```python
from build123d import *

# Parameters (mm, degrees)
F1_DEPTH = 6
F5_DEPTH = 9
F2_R     = 2.05
F6_DEPTH = 13
F2_R_2   = 3.5
F7_DEPTH = 2
F8_DEPTH = 2
F9_R     = 4


with BuildPart() as f1:
    # F0 (on Top) → F1 (new body, symmetric)
    with BuildSketch(Plane.XY):
        with BuildLine():
            ThreePointArc((-22.449944, 1.5), (22.5, 0), (-22.449944, -1.5))
            Line((-22.449944, -1.5), (-41.327112, -1.5))
            Line((-41.327112, -1.5), (-41.327112, -6.5))
            Line((-41.327112, -6.5), (-25.690465, -6.5))
            ThreePointArc((-25.690465, -6.5), (1.022294, -26.480274), (26.11513, -4.5))
            Line((26.11513, -4.5), (40.11513, -4.5))
            Line((40.11513, -4.5), (40.11513, 4.5))
            Line((40.11513, 4.5), (26.11513, 4.5))
            ThreePointArc((26.11513, 4.5), (1.022294, 26.480274), (-25.690465, 6.5))
            Line((-25.690465, 6.5), (-41.327112, 6.5))
            Line((-41.327112, 6.5), (-41.327112, 1.5))
            Line((-41.327112, 1.5), (-22.449944, 1.5))
        make_face()
    extrude(amount=F1_DEPTH, both=True)

    # F4 (on face) → F5 (cut, through all)
    with BuildSketch(Plane.XZ.offset(4.5)):
        with BuildLine():
            ThreePointArc((38.61513, -6), (37.55447, -5.56066), (37.11513, -4.5))
            Line((37.11513, -4.5), (37.11513, 1.5))
            ThreePointArc((37.11513, 1.5), (36.529343, 2.914214), (35.11513, 3.5))
            Line((35.11513, 3.5), (29.61513, 3.5))
            ThreePointArc((29.61513, 3.5), (28.200916, 2.914214), (27.61513, 1.5))
            Line((27.61513, 1.5), (27.61513, -1.5))
            ThreePointArc((27.61513, -1.5), (28.200916, -2.914214), (29.61513, -3.5))
            ThreePointArc((29.61513, -3.5), (31.029343, -2.914214), (31.61513, -1.5))
            Line((31.61513, -1.5), (31.61513, 0))
            ThreePointArc((31.61513, 0), (32.05447, 1.06066), (33.11513, 1.5))
            ThreePointArc((33.11513, 1.5), (34.17579, 1.06066), (34.61513, 0))
            Line((34.61513, 0), (34.61513, -4))
            ThreePointArc((34.61513, -4), (34.029343, -5.414214), (32.61513, -6))
            Line((32.61513, -6), (34.61513, -6))
            Line((34.61513, -6), (37.11513, -6))
            Line((37.11513, -6), (38.61513, -6))
        make_face()
    extrude(amount=-F5_DEPTH, mode=Mode.SUBTRACT)

    # F2 (on face) → F6 (cut, through all)
    with BuildSketch(Plane.XZ.offset(6.5)):
        with Locations((-33.508788, 0)):
            Circle(F2_R)
    extrude(amount=-F6_DEPTH, mode=Mode.SUBTRACT)

    # F2 (on face) → F7 (cut)
    with BuildSketch(Plane.XZ.offset(6.5)):
        with Locations((-33.508788, 0)):
            Circle(F2_R_2)
        with Locations((-33.508788, 0)):
            Circle(F2_R, mode=Mode.SUBTRACT)
    extrude(amount=-F7_DEPTH, mode=Mode.SUBTRACT)

    # F3 (on face) → F8 (cut)
    with BuildSketch(Plane(origin=(0, 6.5, 0), x_dir=(-1, 0, 0), z_dir=(0, 1, 0))):
        Polygon((31.258788, -3.897114), (35.758788, -3.897114), (38.008788, 0), (35.758788, 3.897114), (31.258788, 3.897114), (29.008788, 0), align=None)
    extrude(amount=-F8_DEPTH, mode=Mode.SUBTRACT)

    # F9
    f9_edges = [f1.edges().sort_by_distance(p)[0] for p in [
        (-41.327112, -4, 6),
        (-41.327112, 4, 6),
        (-41.327112, 4, -6),
        (-41.327112, -4, -6),
        (40.11513, 0, 6),
    ]]
    fillet(f9_edges, radius=F9_R)


solid = f1.part
```
CAD build for the part. Positions are in the model's coordinates, mm. A direction names the side the tool comes from. Round coordinates to 2 decimals unless told otherwise and drop trailing zeros. Loops run counter-clockwise (first coordinate to the right, second up) from the corner with the lowest first, then second, coordinate; pieces in that order, holes last. Notation, with made-up numbers: M -20.5,42.25 L 2.5,42.25 A27 ccw 2.5,75.25 Z; hole C 8.5,-8.75 d4. An arc over 180 degrees is marked long. Use a Markdown table: item, result. Add a question column.
(1) Cut at A-A (x = 0). Give the cut face in (y, z).
(2) Cut at C-C (y = 0). Give the cut face in (x, z), and give its area (3 significant figures).
(3) Drill centre lines: line 1 (Y direction, x = -0.5, z = -2.25); line 2 (Y direction, x = -1.5, z = -1.5); line 3 (X direction, y = -5.5, z = -5). Where is each one in solid material? Low to high.
(4) Cut at B-B (y = 10). Give the cut face in (x, z), and give its area (3 significant figures).
(5) Which spindle directions (+Z, -Z, +X, -X, +Y, -Y) get a long thin tool onto all of the face, cutting with end or side? Do faces 1 (the face through (-33.4, 6.5, 4.1)), 2 (the face through (36.545, -0.063, 2.899)), 3 (the face through (33, -4.5, 0)), 4 (the face through (-34, 6, 3.897)). Say none if no direction does.
(6) Flat gauge pins, fed straight in: pin 1 (3.5 mm diameter, centred on x = -33, z = 1, fed in from +Y); pin 2 (6 mm diameter, centred on x = 31.5, z = 1, fed in from -Y); pin 3 (3 mm diameter, centred on y = -9, z = -3.5, fed in from +X). Where does each tip first touch, or does it go through?
(7) Pull direction Z, two halves, no side cores. Call faces 5 (the face through (-30.15, 5.51, 1.98)), 6 (the face through (-40.124, -4.035, -4.859)), 7 (the face through (-23, 2, 6)): +Z half, -Z half, draft (parallel to the pull), parting line (faces both ways), or undercut.
Geometry says:
| question | item | result |
|---|---|---|
| 1 | outline | M -26.5,-6 L -22.5,-6 L -22.5,6 L -26.5,6 Z; M 22.5,-6 L 26.5,-6 L 26.5,6 L 22.5,6 Z |
| 2 | outline | M 22.5,-6 L 32.62,-6 A2 ccw 34.62,-4 L 34.62,0 A1.5 ccw 33.12,1.5 A1.5 ccw 31.62,0 L 31.62,-1.5 A2 cw 29.62,-3.5 A2 cw 27.62,-1.5 L 27.62,1.5 A2 cw 29.62,3.5 L 35.12,3.5 A2 cw 37.12,1.5 L 37.12,-4.5 A1.5 ccw 38.62,-6 L 40.12,-6 L 40.12,2 A4 ccw 36.12,6 L 22.5,6 Z |
| 2 | area | 151 mm² |
| 3 | line 1 | y = -26.5 to -22.49, 22.49 to 26.5 |
| 3 | line 2 | y = -26.46 to -22.45, 22.45 to 26.46 |
| 3 | line 3 | x = -39.97 to -21.82, 21.82 to 25.92 |
| 4 | outline | M -24.54,-6 L -20.16,-6 L -20.16,6 L -24.54,6 Z; M 20.16,-6 L 24.54,-6 L 24.54,6 L 20.16,6 Z |
| 4 | area | 105 mm² |
| 5 | face 1 | +Z, -Z, -X, +Y |
| 5 | face 2 | -Z, +Y, -Y |
| 5 | face 3 | +Z, -Z, +X, -Y |
| 5 | face 4 | +Y |
| 6 | pin 1 | stops at y = 4.5 |
| 6 | pin 2 | stops at y = -4.5 |
| 6 | pin 3 | stops at x = 25.42 |
| 7 | face 5 | undercut |
| 7 | face 6 | -Z half |
| 7 | face 7 | +Z half |
